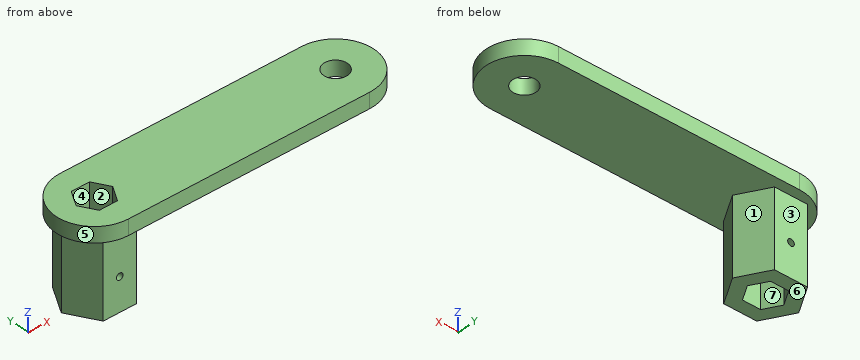
Autodesk Inventor part; units mm, degrees
ref_plane "Work Plane4" through (0, 0, 3) normal (0, 0, 1) x (1, 0, 0)
ref_plane "YZ Plane" through (0, 0, 0) normal (1, 0, 0) x (0, 1, 0)
ref_plane "XZ Plane" through (0, 0, 0) normal (0, 1, 0) x (-1, 0, 0)
ref_plane "Work Plane4" through (0, 0, 3) normal (0, 0, 1) x (1, 0, 0)
sketch "Sketch3" plane through (0, 0, 3) normal (0, 0, 1) x (1, 0, 0)
  circle A0 centre (47, 0) radius 2.3
  circle A1 centre (0, 0) radius 7.5
  circle A2 centre (47, 0) radius 7.5
  line L0 (0, -7.5) -> (47, -7.5)
  line L1 (47, 0) -> (12.3969, 0) construction
  line L2 (0, 7.5) -> (47, 7.5)
  point P0 (0, 0)
  dimension "d13" = 15
  dimension "d5" = 4.6
  dimension "d14" = 47
extrude "Extrusion5" add sketch "Sketch3" along normal blind 3
sketch "Sketch6" plane through (0, 0, 3) normal (0, 0, -1) x (-1, 0, 0)
  arc A0 (0, -7.5) -> (0, 7.5) centre (0, 0) ccw
  line L0 (0, 0) -> (3.1, 0) construction
  line L1 (0, 0) -> (1.55, 2.6847) construction
  line L2 (0, 0) -> (-1.55, 2.6847) construction
  line L3 (0, 0) -> (-3.1, 0) construction
  line L4 (0, 0) -> (-1.55, -2.6847) construction
  line L5 (0, 0) -> (1.55, -2.6847) construction
  line L6 (-1.55, 2.6847) -> (1.55, 2.6847) construction
  line L7 (1.55, 2.6847) -> (3.1, 0) construction
  line L8 (3.1, 0) -> (1.55, -2.6847) construction
  line L9 (1.55, -2.6847) -> (-1.55, -2.6847) construction
  line L10 (-1.55, -2.6847) -> (-3.1, 0) construction
  line L11 (-3.1, 0) -> (-1.55, 2.6847) construction
  line L12 (3.5619, 0) -> (1.7809, 3.0847)
  line L13 (1.7809, 3.0847) -> (-1.7809, 3.0847)
  line L14 (-1.7809, 3.0847) -> (-3.5619, 0)
  line L15 (-3.5619, 0) -> (-1.7809, -3.0847)
  line L16 (-1.7809, -3.0847) -> (1.7809, -3.0847)
  line L17 (1.7809, -3.0847) -> (3.5619, 0)
  line L18 (3.2243, 5.5847) -> (6.4486, 0)
  line L19 (6.4486, 0) -> (3.2243, -5.5847)
  line L20 (3.2243, -5.5847) -> (-3.2243, -5.5847)
  line L21 (-3.2243, -5.5847) -> (-6.4486, 0)
  line L22 (-6.4486, 0) -> (-3.2243, 5.5847)
  line L23 (-3.2243, 5.5847) -> (3.2243, 5.5847)
  point P0 (0, 0)
  dimension "d17" = 3.1
  dimension "d20" = 360
  dimension "d22" = 0.4
  dimension "d23" = 2.5
extrude "Extrusion6" add sketch "Sketch6" along normal blind 15
sketch "Sketch7" plane through (0, 0, 3) normal (0, 0, -1) x (-1, 0, 0)
  line L0 (3.5619, 0) -> (1.7809, 3.0847)
  line L1 (1.7809, 3.0847) -> (-1.7809, 3.0847)
  line L2 (-1.7809, 3.0847) -> (-3.5619, 0)
  line L3 (-3.5619, 0) -> (-1.7809, -3.0847)
  line L4 (-1.7809, -3.0847) -> (1.7809, -3.0847)
  line L5 (1.7809, -3.0847) -> (3.5619, 0)
  point P0 (0, 0)
extrude "Extrusion7" cut sketch "Sketch7" against normal blind 15
sketch "Sketch8" plane through (-3.2243, 5.5847, 3) normal (0, 1, 0) x (1, 0, 0)
  line L0 (6.4486, 0) -> (0, 0)
  line L1 (6.4486, 0) -> (6.4486, 15)
  line L2 (0, 15) -> (6.4486, 15)
  line L3 (0, 0) -> (0, 15)
  line L4 (0, 0) -> (0, 15)
  line L5 (1.4434, 15) -> (5.0053, 15)
  line L6 (3.2243, 0) -> (3.2243, -3)
  line L7 (3.2243, 15) -> (3.2243, 0) construction
  circle A0 centre (3.2243, 8.5) radius 0.65
  line L8 (-4.2757, -3) -> (3.2243, -3)
  point P0 (3.2243, 3)
  dimension "d29" = 1.3
  dimension "d30" = 11.5
extrude "Extrusion8" cut sketch "Sketch8" against normal blind 15 contours A0
properties part number "Acople_TransPot"
Check sheet for the modelled part. Datum: model origin and axes. Units: mm. Face numbers are marked on the shaded views. A direction names the side the tool comes from. Give positions to 0.01 mm unless a question says otherwise; leave off trailing zeros. Write each loop counter-clockwise with the first axis right and the second up, starting at its lowest first coordinate (ties: lowest second). Pieces come first, ordered by that corner, then holes. Notation, with made-up numbers: M 53,-26 L 76,-26 A19 ccw 76,-13 Z; hole C -40,24.25 d11. An arc over 180 degrees is marked long. Use one line per item in the form item = value.
(1) Material ranges on line 1 along Z through (x, y) = (0, -3.75); line 2 along Y through (x, z) = (-1, -9.5); line 3 along Z through (x, y) = (34.5, 1.5), recorded low to high.
Answer block:
line_1 = -12 to -6.15, -4.85 to 6
line_2 = -5.58 to -3.08, 3.08 to 5.58
line_3 = 3 to 6
(2) Draft check along X on the marked faces 4, 5, 6 and 7. Enter one of: pulls with the +X half, pulls with the -X half, needs draft (parallel to the pull), parting line crosses it, or undercut.
Answer block:
face_4 = undercut
face_5 = pulls with the -X half
face_6 = needs draft
face_7 = undercut
(3) Section check C-C on y = -0.75. Record the boundary of the cut face in (x, z).
Answer block:
outline = M -7.46,3 L -6.02,3 L -6.02,-12 L -3.13,-12 L -3.13,6 L -7.46,6 Z; M 3.13,-12 L 6.02,-12 L 6.02,3 L 44.83,3 L 44.83,6 L 3.13,6 Z; M 49.17,3 L 54.46,3 L 54.46,6 L 49.17,6 Z
(4) Tool access check on the marked faces 1, 2 and 3. Record the directions out of +Z, -Z, +X, -X, +Y, -Y that give a thin tool (end or side, any length) a straight path to the whole face; none if there is none.
Answer block:
face_1 = -Z, +X, +Y
face_2 = +Z, -Z
face_3 = -Z, +X, -X, +Y
(5) Section check D-D on z = 4.25. Record the boundary of the cut face in (x, y), plus the area to 3 significant figures.
Answer block:
outline = M 0,-7.5 L 47,-7.5 A7.5 ccw 47,7.5 L 0,7.5 A7.5 ccw Z; hole M -3.56,0 L -1.78,-3.08 L 1.78,-3.08 L 3.56,0 L 1.78,3.08 L -1.78,3.08 Z; hole C 47,0 d4.6
area = 832 mm2
(6) Section check A-A on z = -8.75. Record the boundary of the cut face in (x, y), plus the area to 3 significant figures.
Answer block:
outline = M -6.45,0 L -3.22,-5.58 L 3.22,-5.58 L 6.45,0 L 3.22,5.58 L -3.22,5.58 Z; hole M -3.56,0 L -1.78,-3.08 L 1.78,-3.08 L 3.56,0 L 1.78,3.08 L -1.78,3.08 Z
area = 75.1 mm2
(7) Section check B-B on z = -5.5. Record the boundary of the cut face in (x, y), plus the area to 3 significant figures.
Answer block:
outline = M -6.45,0 L -3.22,-5.58 L -0.65,-5.58 L -0.65,-3.08 L -1.78,-3.08 L -3.56,0 L -1.78,3.08 L -0.65,3.08 L -0.65,5.58 L -3.22,5.58 Z; M 0.65,-5.58 L 3.22,-5.58 L 6.45,0 L 3.22,5.58 L 0.65,5.58 L 0.65,3.08 L 1.78,3.08 L 3.56,0 L 1.78,-3.08 L 0.65,-3.08 Z
area = 68.6 mm2
(8) Depth check by flat-ended pin: P1, Ø7, axis at x = -1.5, z = -2.5, coming from the -Y side; P2, Ø4.5, axis at x = 27, y = -2.5, coming from the -Z side; P3, Ø3, axis at x = 1.5, z = -5, coming from the +Y side. Enter the tip coordinate at first touch or a pass-through.
Answer block:
P1 = -5.58
P2 = 3
P3 = 5.58
